```python
from build123d import *

# Parameters (mm, degrees)
BOSS_EXTRUDE1_DEPTH     = 10
BOSS_EXTRUDE2_DEPTH     = 30
BOSS_EXTRUDE3_DEPTH     = 4
CHAMFER1_SIZE           = 2
CUT_EXTRUDE1_DEPTH      = 78.548774974
CUT_EXTRUDE1_DEPTH_BACK = 78.548774974
SKETCH5_R               = 2
BOSS_EXTRUDE4_START     = -4
SKETCH6_R               = 2
BOSS_EXTRUDE4_DEPTH     = 4
FILLET1_R               = 10


with BuildPart() as part:
    # Sketch1 → Boss-Extrude1 (new body)
    with BuildSketch(Plane(origin=(0, 0, 0), x_dir=(1, 0, 0), z_dir=(0, 1, 0))):
        with BuildLine():
            ThreePointArc((-25.25, -43.734282891), (0, -50.5), (25.25, -43.734282891))
            Line((25.25, -43.734282891), (27.25, -47.198384506))
            ThreePointArc((27.25, -47.198384506), (0, -54.5), (-27.25, -47.198384506))
            Line((-27.25, -47.198384506), (-25.25, -43.734282891))
        make_face()
    extrude(amount=BOSS_EXTRUDE1_DEPTH)



with BuildPart() as body_2:
    # Sketch3 → Boss-Extrude2 (new body)
    with BuildSketch(Plane.XZ):
        with BuildLine():
            Line((-30.25, 52.394536929), (-28.75, 49.796460718))
            ThreePointArc((-28.75, 49.796460718), (0, 57.5), (28.75, 49.796460718))
            Line((28.75, 49.796460718), (30.25, 52.394536929))
            ThreePointArc((30.25, 52.394536929), (0, 60.5), (-30.25, 52.394536929))
        make_face()
    extrude(amount=-BOSS_EXTRUDE2_DEPTH)


with BuildPart() as part_1:
    add(part.part)

    add(body_2.part)  # Boss-Extrude3 merges body 2
    # Sketch4 → Boss-Extrude3 (add)
    with BuildSketch(Plane.XZ):
        with BuildLine():
            ThreePointArc((-24.25, 42.002232084), (0, 48.5), (24.25, 42.002232084))
            ThreePointArc((24.25, 42.002232084), (33.812177826, 44.56440991), (31.25, 54.126587737))
            ThreePointArc((31.25, 54.126587737), (0, 62.5), (-31.25, 54.126587737))
            ThreePointArc((-31.25, 54.126587737), (-33.812177826, 44.56440991), (-24.25, 42.002232084))
        make_face()
    extrude(amount=BOSS_EXTRUDE3_DEPTH)

    # Chamfer1
    chamfer1_edges = [part_1.edges().sort_by_distance(p)[0] for p in [
        (0, 0, 60.5),
        (0, 0, 50.5),
    ]]
    chamfer(chamfer1_edges, length=CHAMFER1_SIZE - 0.0001)  # a hair under: the kernel refuses the full size

    # Sketch5 → Cut-Extrude1 (cut, two sides: drawn at the far end of the back side and taken through both)
    with BuildSketch(Plane.XY.offset(-CUT_EXTRUDE1_DEPTH_BACK)):
        with Locations(Location((0, 16, 0), (0, 0, 180))):
            Circle(SKETCH5_R)
        with Locations(Location((-20, 16, 0), (0, 0, 180))):
            Circle(SKETCH5_R)
        with Locations(Location((20, 16, 0), (0, 0, 180))):
            Circle(SKETCH5_R)
    extrude(amount=CUT_EXTRUDE1_DEPTH + CUT_EXTRUDE1_DEPTH_BACK, mode=Mode.SUBTRACT)

    # Sketch6 → Boss-Extrude4 (add)
    # profile 1 of 2: a face of its own
    with BuildSketch(Plane.XZ.offset(4).offset(BOSS_EXTRUDE4_START)):
        with BuildLine():
            Line((20.953972553, 58.882773663), (24.414654978, 71.798216302))
            ThreePointArc((24.414654978, 71.798216302), (24.468385119, 73.111891055), (23.955219754, 74.322382523))
            ThreePointArc((23.955219754, 74.322382523), (20.546663808, 76.681193258), (16.415362401, 76.342681212))
            ThreePointArc((16.415362401, 76.342681212), (15.365702425, 75.550947532), (14.755396715, 74.386406753))
            Line((14.755396715, 74.386406753), (11.29471429, 61.470964114))
            ThreePointArc((11.29471429, 61.470964114), (16.176190319, 60.370364143), (20.953972553, 58.882773663))
        make_face()
        with Locations(Location((18.213190451, 67.972552131, 0), (0, 0, 270))):
            Circle(SKETCH6_R, mode=Mode.SUBTRACT)
    # profile 2 of 2: a face of its own
    with BuildSketch(Plane.XZ.offset(4).offset(BOSS_EXTRUDE4_START)):
        with BuildLine():
            Line((-20.953972553, 58.882773663), (-24.414654978, 71.798216302))
            ThreePointArc((-24.414654978, 71.798216302), (-24.468385119, 73.111891055), (-23.955219754, 74.322382523))
            ThreePointArc((-23.955219754, 74.322382523), (-20.546663808, 76.681193258), (-16.415362401, 76.342681212))
            ThreePointArc((-16.415362401, 76.342681212), (-15.365702425, 75.550947532), (-14.755396715, 74.386406753))
            Line((-14.755396715, 74.386406753), (-11.29471429, 61.470964114))
            ThreePointArc((-11.29471429, 61.470964114), (-16.176190319, 60.370364143), (-20.953972553, 58.882773663))
        make_face()
        with Locations(Location((-18.213190451, 67.972552131, 0), (0, 0, 270))):
            Circle(SKETCH6_R, mode=Mode.SUBTRACT)
    extrude(amount=BOSS_EXTRUDE4_DEPTH)

    # Fillet1
    fillet1_edges = [part_1.edges().sort_by_distance(p)[0] for p in [
        (-11.29471429, -2, 61.470964114),
        (-20.953972553, -2, 58.882773663),
        (20.953972553, -2, 58.882773663),
        (11.29471429, -2, 61.470964114),
    ]]
    fillet(fillet1_edges, radius=FILLET1_R)


solid = part_1.part
```
Here's how the part is built. I have some questions about the finished solid (model axes, mm). A direction names the side the tool comes from. Coordinates: 2 decimals unless noted, no trailing zeros. Order: outer loops, then holes, each group sorted by start corner. A loop starts at its lowest first (then second) coordinate and runs counter-clockwise, first axis right, second up. Notation, with made-up numbers: (45, -6) - (76, -6) arc R15 cw to (76, 1) - close; hole circle Ø9 at (0.5, 49). An arc over 180 degrees is marked (long way). One line per question, with ' | ' between items. Start each with the question number.
1. I'm going to push flat-ended pins straight in: pin 1 Ø6.5 at (x, y) = (0, 16) entering from +Z; pin 2 Ø3 at (x, y) = (15, 13) entering from +Z; pin 3 Ø4 at (x, z) = (-27.5, 45.5) entering from +Y; pin 4 Ø3.5 at (x, y) = (-20, 16) entering from +Z. Where does each tip first touch, or does it pass through?
2. If we section it at B-B (z = 63.5): Write out the boundary of the cut face in (x, y), and give its area (3 significant figures).
3. Please list where these lines run through material, in increasing order: line 1 along Y through (x, z) = (-20, 56.8); line 2 along Y through (x, z) = (-13.5, 61.5); line 3 along Y through (x, z) = (6, 51). Write a range as [from, to].
4. If we mould it in two halves opening along Y, with no side actions, what happens to faces 6 (the conical face through (0.4, 1.7, 60.8)), 7 (the flat face through (29.427, 14.79, 50.969)), 8 (the cylindrical face through (21.474, 14.648, 55.404))? For each: released by +Y, released by -Y, zero draft, split by the parting line, or undercut.
5. If we section it at C-C (y = 22.5): Write out the boundary of the cut face in (x, z), and give its area (3 significant figures).
6. Which directions (+Z, -Z, +X, -X, +Y, -Y) give clear straight access to the entire face, cutting with the end or side of a thin tool? Please do faces 1 (the cylindrical face through (0.4, 12.7, 60.5)), 2 (the flat face through (23.8, -2, 69.5)), 3 (the cylindrical face through (-0.4, 5.9, 50.5)), 4 (the flat face through (-23.8, -2, 69.5)), 5 (the flat face through (-14.15, -1.97, 72.13)).
Model answer:
1) pin 1: stops at z = 60.5 | pin 2: stops at z = 58.97 | pin 3: stops at y = 10 | pin 4: passes through
2) outline: (-22.91, -4) - (-8.44, -4) - (-8.44, 0) - (-22.91, 0) - close; (8.44, -4) - (22.91, -4) - (22.91, 0) - (8.44, 0) - close | area: 116 mm²
3) line 1: y = [-4, 14], [18, 30] | line 2: y = [-4, 0] | line 3: y = [-4, 10]
4) face 6: released by +Y | face 7: zero draft | face 8: undercut
5) outline: (-30.25, 52.39) - (-28.75, 49.8) arc R57.5 cw to (28.75, 49.8) - (30.25, 52.39) arc R60.5 ccw to start | area: 185 mm²
6) face 1: +Z, +Y | face 2: +X, +Y, -Y | face 3: -Z, +Y | face 4: -X, +Y, -Y | face 5: +Z, +Y, -Y
